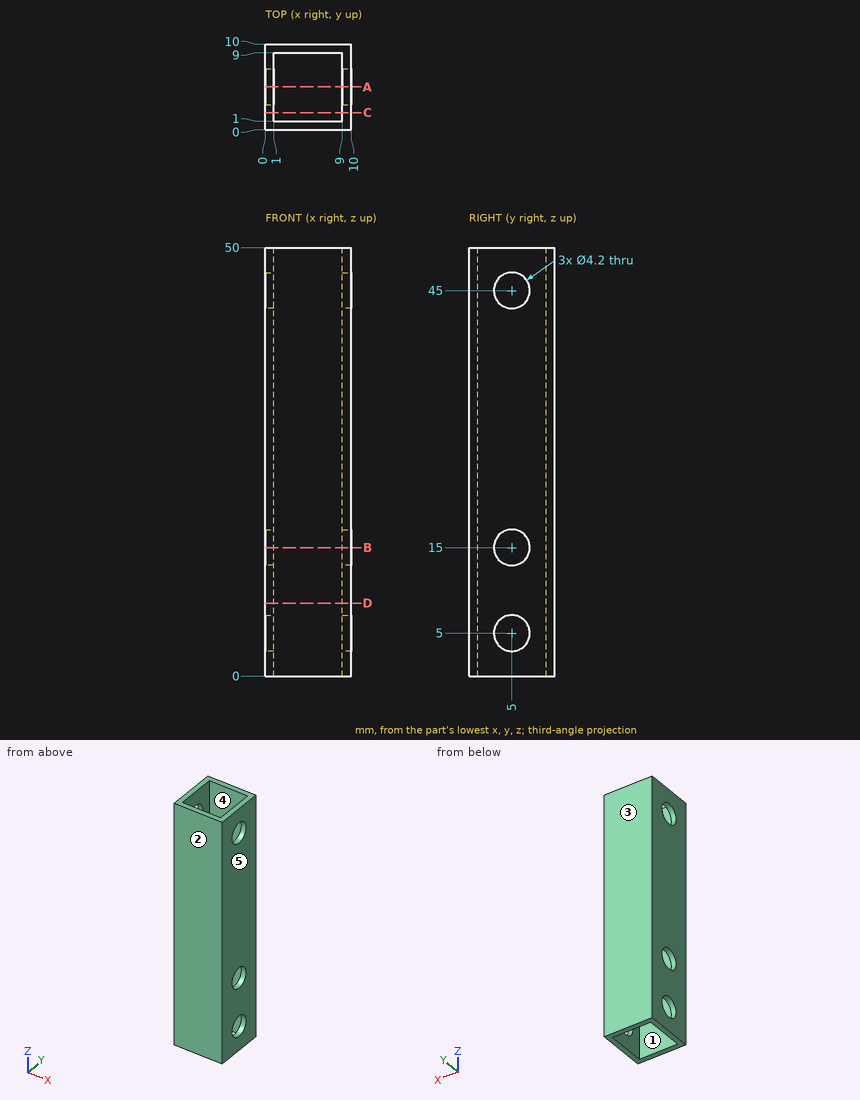
Verification items for this drawing (mm, ordinates from the low corner). A direction names the side the tool comes from. Coordinates: 2 decimals unless noted, no trailing zeros. Write each loop counter-clockwise with the first axis right and the second up, starting at its lowest first coordinate (ties: lowest second). Pieces come first, ordered by that corner, then holes. Notation, with made-up numbers: M 21.5,-30.5 L 32.5,-30.5 A18 cw 32.5,-9.5 Z; hole C 19,31.25 d1. An arc over 180 degrees is marked long. Answer as a JSON object with one key per item and string values.
1. Section check C-C, the plane y = 2. Enter the section's corners in (x, z), plus the area to 3 significant figures.
Answers below:
{"outline": "M 0,0 L 1,0 L 1,50 L 0,50 Z; M 9,0 L 10,0 L 10,50 L 9,50 Z", "area": "100 mm²"}
2. Tool access check on the marked faces 1 and 2. Record the directions out of +Z, -Z, +X, -X, +Y, -Y that give a thin tool (end or side, any length) a straight path to the whole face; none if there is none.
Answers below:
{"face 1": "+Z, -Z", "face 2": "+Z, -Z, +X, -X, -Y"}
3. Draft check along X on the marked faces 3, 4 and 5. Enter one of: released by +X, released by -X, zero draft, split by the parting line, or undercut.
Answers below:
{"face 3": "zero draft", "face 4": "undercut", "face 5": "released by +X"}
4. Section check B-B, the plane z = 15. Enter the section's corners in (x, y), plus the area to 3 significant figures.
Answers below:
{"outline": "M 0,0 L 10,0 L 10,2.9 L 9,2.9 L 9,1 L 1,1 L 1,2.9 L 0,2.9 Z; M 0,7.1 L 1,7.1 L 1,9 L 9,9 L 9,7.1 L 10,7.1 L 10,10 L 0,10 Z", "area": "27.6 mm²"}
5. Section check A-A, the plane y = 5. Give the number of separate pieces and of enclosed holes in the cut face, plus the area to 3 significant figures.
Answers below:
{"separate pieces": "8", "enclosed holes": "0", "area": "74.8 mm²"}
6. Go/stop test with a flat-tipped pin: pin 1 Ø2.5 at (y, z) = (5, 45) entering from +X. Record where the tip stops, or that it passes through.
Answers below:
{"pin 1": "passes through"}
7. Scan lines: L1, parallel to Y at x = 8, z = 38; L2, parallel to Y at x = 9.2, z = 45. Record each from-to range of solid material in increasing order.
Answers below:
{"L1": "y = 0 to 1, 9 to 10", "L2": "y = 0 to 2.9, 7.1 to 10"}
8. Section check D-D, the plane z = 8.5. Enter the section's corners in (x, y), plus the area to 3 significant figures.
Answers below:
{"outline": "M 0,0 L 10,0 L 10,10 L 0,10 Z; hole M 1,1 L 9,1 L 9,9 L 1,9 Z", "area": "36.0 mm²"}
